from build123d import *

# Parameters (mm, degrees)
SKETCH3_W            = 50
SKETCH3_H            = 27
BOSS_EXTRUDE1_DEPTH  = 5
BOSS_EXTRUDE2_DEPTH  = 5
M5_CLEARANCE_HOLE1_D = 5.3
FILLET1_R            = 6
M5_CLEARANCE_HOLE2_D = 5.3
SKETCH11_R           = 7
BOSS_EXTRUDE3_DEPTH  = 4.1
CUT_EXTRUDE1_DEPTH   = 23
FILLET2_R            = 3
FILLET3_R            = 1
SKETCH12_W           = 14
SKETCH12_H           = 4.5
BOSS_EXTRUDE4_DEPTH  = 2.5
BOSS_EXTRUDE5_DEPTH  = 2.5
SKETCH14_W           = 10.641777725
SKETCH14_H           = 9.1
BOSS_EXTRUDE6_DEPTH  = 2.5
FILLET4_R            = 1
CUT_EXTRUDE2_DEPTH   = 6
FILLET5_R            = 1


with BuildPart() as part:
    # Sketch3 → Boss-Extrude1 (new body)
    with BuildSketch(Plane.XY):
        with Locations((-63, -14.5)):
            Rectangle(SKETCH3_W, SKETCH3_H)
    extrude(amount=BOSS_EXTRUDE1_DEPTH)

    # Sketch5 → Boss-Extrude2 (add)
    with BuildSketch(Plane.XZ.offset(28)):
        with BuildLine():
            Line((-38, 5), (-77.841460566, 63.448623046))
            ThreePointArc((-77.841460566, 63.448623046), (-97.078370732, 68.348402277), (-104.331234438, 49.86969785))
            Line((-104.331234438, 49.86969785), (-88, 5))
            Line((-88, 5), (-88, 0))
            Line((-88, 0), (-38, 0))
            Line((-38, 0), (-38, 5))
        make_face()
    extrude(amount=-BOSS_EXTRUDE2_DEPTH)

    # M5 Clearance Hole1 (through all)
    with Locations(Plane.XY.offset(5)):
        with Locations((-79, -10), (-47, -10)):
            Hole(M5_CLEARANCE_HOLE1_D / 2)

    # Fillet1
    fillet1_edges = [part.edges().sort_by_distance(p)[0] for p in [
        (-63, -23, 5),
        (-88, -1, 2.5),
        (-38, -1, 2.5),
    ]]
    fillet(fillet1_edges, radius=FILLET1_R)

    # M5 Clearance Hole2 (through all)
    with Locations(Plane(origin=(0, -23, 0), x_dir=(1, 0, 0), z_dir=(0, 1, 0))):
        with Locations((-90.235845126, -55)):
            Hole(M5_CLEARANCE_HOLE2_D / 2)

    # Sketch11 → Boss-Extrude3 (add)
    with BuildSketch(Plane(origin=(0, -23, 0), x_dir=(1, 0, 0), z_dir=(0, 1, 0))):
        with Locations((-90.235845126, -55)):
            Circle(SKETCH11_R)
    extrude(amount=BOSS_EXTRUDE3_DEPTH)

    # Sketch10 → Cut-Extrude1 (cut, through all)
    with BuildSketch(Plane(origin=(0, -23, 0), x_dir=(1, 0, 0), z_dir=(0, 1, 0))):
        Polygon((-92.562566711, -50.97), (-94.889288296, -55), (-92.562566711, -59.03), (-87.909123541, -59.03), (-85.582401957, -55), (-87.909123541, -50.97), align=None)
    extrude(amount=CUT_EXTRUDE1_DEPTH, mode=Mode.SUBTRACT)

    # Fillet2
    fillet2_edges = [part.edges().sort_by_distance(p)[0] for p in [
        (-97.235845126, -23, 55),
    ]]
    fillet(fillet2_edges, radius=FILLET2_R)

    # Fillet3
    fillet3_edges = [part.edges().sort_by_distance(p)[0] for p in [
        (-97.235845126, -18.9, 55),
    ]]
    fillet(fillet3_edges, radius=FILLET3_R)

    # Sketch12 → Boss-Extrude4 (add)
    with BuildSketch(Plane(origin=(0, 0, 0), x_dir=(-1, 0, 0), z_dir=(0, 0, -1))):
        with Locations((63, -10)):
            Rectangle(SKETCH12_W, SKETCH12_H)
    extrude(amount=BOSS_EXTRUDE4_DEPTH)

    # Sketch13 → Boss-Extrude5 (add)
    with BuildSketch(Plane.XZ.offset(28)):
        Polygon((-91.639702343, 15), (-97.639702343, 15), (-101.279404685, 25), (-95.279404685, 25), align=None)
    extrude(amount=-BOSS_EXTRUDE5_DEPTH)

    # Sketch14 → Boss-Extrude6 (add)
    with BuildSketch(Plane(origin=(-81.397119802, 0, -29.626128763), x_dir=(-0.342020143, 0, 0.939692621), z_dir=(-0.939692621, 0, -0.342020143))):
        with Locations((52.811023164, -23.45)):
            Rectangle(SKETCH14_W, SKETCH14_H)
    extrude(amount=BOSS_EXTRUDE6_DEPTH)

    # Fillet4
    fillet4_edges = [part.edges().sort_by_distance(p)[0] for p in [
        (-93.459553514, -25.5, 20),
        (-99.459553514, -25.5, 20),
        (-99.459553514, -18.9, 20),
        (-102.454020461, -18.9, 24.572474821),
        (-98.814318119, -18.9, 14.572474821),
        (-101.808785066, -18.9, 19.144949642),
    ]]
    fillet(fillet4_edges, radius=FILLET4_R)

    # Sketch15 → Cut-Extrude2 (cut, through all)
    with BuildSketch(Plane(origin=(0, -23, 0), x_dir=(1, 0, 0), z_dir=(0, 1, 0))):
        with BuildLine():
            Line((-81.725865086, -17), (-58.2820459, -17))
            Line((-58.2820459, -17), (-78.739044792, -47.011033729))
            ThreePointArc((-78.739044792, -47.011033729), (-83.849487894, -42.541491209), (-90.461814506, -41.001823767))
            Line((-90.461814506, -41.001823767), (-81.725865086, -17))
        make_face()
    extrude(amount=-CUT_EXTRUDE2_DEPTH, mode=Mode.SUBTRACT)

    # Fillet5
    fillet5_edges = [part.edges().sort_by_distance(p)[0] for p in [
        (-90.461814506, -25.5, 41.001823767),
        (-81.725865086, -25.5, 17),
        (-58.2820459, -25.5, 17),
        (-78.739044792, -25.5, 47.011033729),
    ]]
    fillet(fillet5_edges, radius=FILLET5_R)


solid = part.part
Check sheet for the modelled part. Datum: model origin and axes. Units: mm. A direction names the side the tool comes from. Round coordinates to 2 decimals unless told otherwise and drop trailing zeros. Loops run counter-clockwise (first coordinate to the right, second up) from the corner with the lowest first, then second, coordinate; pieces in that order, holes last.
1. Sectioned sample at B-B on x = -74. Record the boundary of the cut face in (y, z).
2. Sectioned sample at D-D on x = -47. Record the boundary of the cut face in (y, z), and give its area (3 significant figures).
3. Set-up check for faces 1 (the flat face through (-93.71, -20.98, 52.96)), 2 (the flat face through (-63, -9, 5)), 3 (the flat face through (-100.6, -18.9, 19.5)), 4 (the cylindrical face through (-59.28, -25.54, 17.55)), 5 (the flat face through (-74, -28, 41)): record each of +Z, -Z, +X, -X, +Y, -Y from which the full face is reachable in a straight line by a thin tool's end or side.
4. Sectioned sample at A-A on y = -10. Record the boundary of the cut face in (x, z).
5. Sectioned sample at C-C on z = 43. Record the boundary of the cut face in (x, y), and give its area (3 significant figures).
6. Scan lines: probe 1 along Y at (x, z) = (-79, 1.45); probe 2 along Y at (x, z) = (-68.5, 42); probe 3 along X at (y, z) = (-25.35, 55). Record each from-to range of solid material in increasing order.
7. Mould release check, pull along Z, two halves, no side actions. Record for faces 6 (the flat face through (-63, -10, -2.5)), 7 (the flat face through (-56, -10, -1)), 8 (the cylindrical face through (-92.763, -25.535, 54.204)), 9 (the cylindrical face through (-96.807, -25.535, 68.484)): released by +Z, released by -Z, zero draft, split by the parting line, or undercut.
8. Gauge pin test, flat ends, axial feed: pin 1 Ø4 at (x, y) = (-84.5, -22.5) entering from +Z; pin 2 Ø0.8 at (y, z) = (-9.5, -1.5) entering from -X; pin 3 Ø1.8 at (x, y) = (-97, -25.5) entering from +Z; pin 4 Ø1.5 at (y, z) = (-15.5, 6.5) entering from -X. Record the tip position at first contact, or that the pin passes through.
Recorded:
1. outline: (-28, 0) - (-1, 0) - (-1, 5) - (-17, 5) arc R6 cw to (-23, 11) - (-23, 17) - (-28, 17) - close; (-28, 40.06) - (-23, 40.06) - (-23, 57.81) - (-28, 57.81) - close
2. outline: (-28, 0) - (-12.65, 0) - (-12.65, 5) - (-17, 5) arc R6 cw to (-23, 11) - (-23, 18.2) - (-28, 18.2) - close; (-7.35, 0) - (-1, 0) - (-1, 5) - (-7.35, 5) - close
2. area: 182 mm2
3. face 1: +Y
3. face 2: +Z, +X, -X, +Y
3. face 3: +Z, -Z, +X, -X, +Y
3. face 4: +Y, -Y
3. face 5: +Z, -Z, +X, -X, -Y
4. outline: (-88, 0) - (-81.65, 0) - (-81.65, 5) - (-88, 5) - close; (-76.35, 0) - (-70, 0) - (-70, -2.5) - (-56, -2.5) - (-56, 0) - (-49.65, 0) - (-49.65, 5) - (-76.35, 5) - close; (-44.35, 0) - (-38, 0) - (-38, 5) - (-44.35, 5) - close
5. outline: (-101.83, -28) - (-83.02, -28) - (-83.02, -23) - (-101.83, -23) - close; (-76, -28) - (-63.9, -28) - (-63.9, -23) - (-76, -23) - close
5. area: 155 mm2
6. probe 1: y = -28 to -12.65, -7.35 to -1
6. probe 2: y = -28 to -23
6. probe 3: x = -105.24 to -92.89, -87.59 to -72.08
7. face 6: released by -Z
7. face 7: zero draft
7. face 8: undercut
7. face 9: split by the parting line
8. pin 1: stops at z = 69.51
8. pin 2: stops at x = -70
8. pin 3: stops at z = 68.81
8. pin 4: passes through
